The drawing under review shows one solid part. Ordinate dimensions are in mm from its lowest x, y, z. A direction names the side the tool comes from. Give positions to 0.01 mm unless a question says otherwise; leave off trailing zeros. Order: outer loops, then holes, each group sorted by start corner. A loop starts at its lowest first (then second) coordinate and runs counter-clockwise, first axis right, second up. Notation, with made-up numbers: (51.25, -39) - (110.25, -39) arc R13 ccw to (110.25, -16) - close; hole circle Ø8 at (-36.5, -38.75). An arc over 180 degrees is marked (long way). Answer as a JSON object with one key per item and string values. Group by question number.
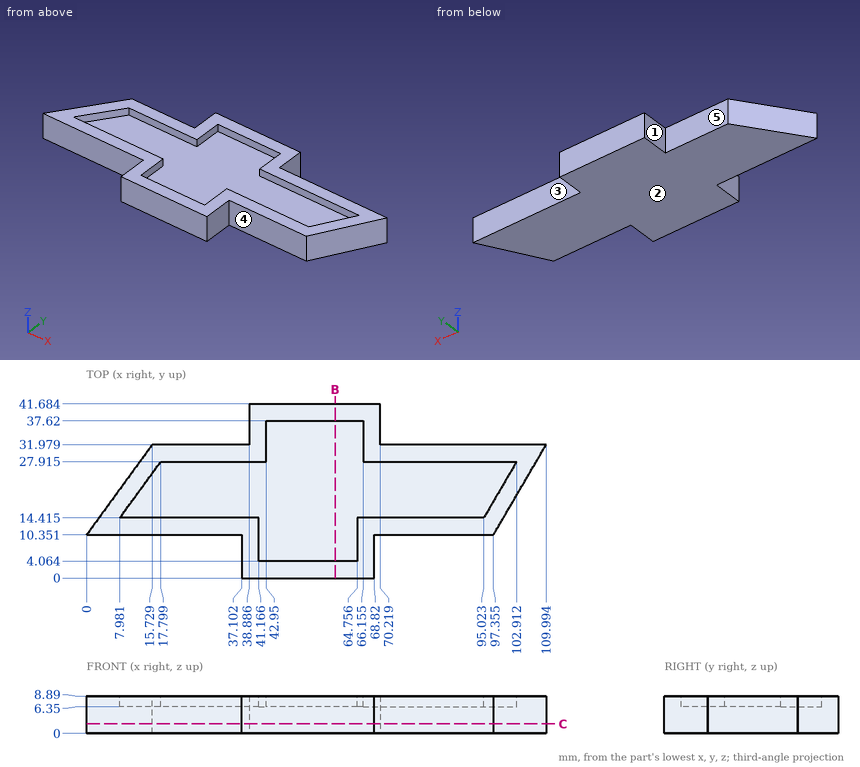
1) Consider section C-C (z = 2.25). Give the boundary of the cut face in (x, y) (1 decimal).
2) For the marked faces 3, 4 and 5, list the 3-axis set-ups (+Z, -Z, +X, -X, +Y, -Y) from which the entire face can be reached by the end or side of a thin tool; tool diameter is ignored.
3) Consider section B-B (x = 59.5). Give the boundary of the cut face in (y, z), plus the area to 3 significant figures.
4) For pin 1 (3 mm diameter, centred on y = 31.5, z = 7.5, fed in from +X); pin 2 (17 mm diameter, centred on x = 56, y = 21.5, fed in from +Z); pin 3 (0.8 mm diameter, centred on y = 11.5, z = 8, fed in from +X); pin 4 (2 mm diameter, centred on x = 92, y = 8.5, fed in from -Z), all flat-tipped, find the tip position at first contact; note any pin that passes through.
5) For line 1 (Y direction, x = 52, z = 7.25); line 2 (Y direction, x = 69.5, z = 6.75) (1 decimal); line 3 (Y direction, x = 71.5, z = 5.75), list the stretches that pass through material, from the lowest coordinate up.
6) Mouldability with a two-part tool opening along Z and no side actions: class the marked faces 1 and 2 as released by +Z, released by -Z, zero draft, split by the parting line, or undercut.
Result set:
{
 "1": {"outline": "(0, 10.4) - (37.1, 10.4) - (37.1, 0) - (68.8, 0) - (68.8, 10.4) - (97.4, 10.4) - (110, 32) - (70.2, 32) - (70.2, 41.7) - (38.9, 41.7) - (38.9, 32) - (15.7, 32) - close"},
 "2": {"face 3": "+Z, -Z, +X, +Y", "face 4": "+Z, -Z, +X, -Y", "face 5": "+Z, -Z, -X, +Y"},
 "3": {"outline": "(0, 0) - (41.68, 0) - (41.68, 8.89) - (37.62, 8.89) - (37.62, 6.35) - (4.06, 6.35) - (4.06, 8.89) - (0, 8.89) - close", "area": "285 mm2"},
 "4": {"pin 1": "stops at x = 109.99", "pin 2": "stops at z = 6.35", "pin 3": "stops at x = 98.26", "pin 4": "passes through"},
 "5": {"line 1": "y = 0 to 4.06, 37.62 to 41.68", "line 2": "y = 10.4 to 14.4, 27.9 to 41.7", "line 3": "y = 10.35 to 31.98"},
 "6": {"face 1": "zero draft", "face 2": "released by -Z"}
}
